Print and shaded views of the part. All mm, measured from the part's lowest x, y and z. A direction names the side the tool comes from. Coordinates: 2 decimals unless noted, no trailing zeros. Loops run counter-clockwise (first coordinate to the right, second up) from the corner with the lowest first, then second, coordinate; pieces in that order, holes last. Notation, with made-up numbers: M 17,65.5 L 23,65.5 A20 cw 23,98.5 Z; hole C 44,30.5 d6. An arc over 180 degrees is marked long. Answer as CSV lines item,"result". Start each with the question number.
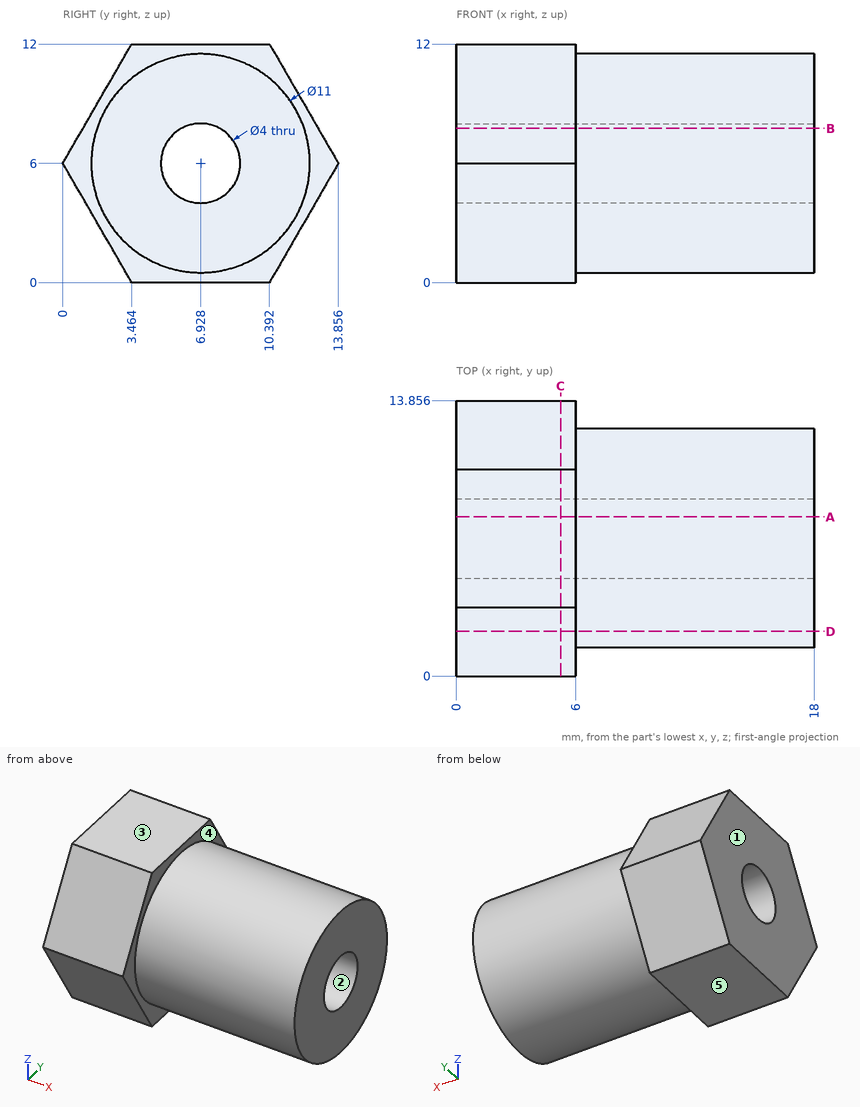
Q1. Two-plate mould, pull along Z, no slides. Class the marked faces 1, 2 and 3: +Z half, -Z half, draft (parallel to the pull), parting line (faces both ways), or undercut.
Q2. Wall check: L1, parallel to Y at x = 12.5, z = 6; L2, parallel to X at y = 12.75, z = 5.25; L3, parallel to Z at x = 10.5, y = 5.75 (1 decimal). Give the ranges that are in metal, low to high.
Q3. Flat gauge pins, fed straight in: P1, Ø3.5, axis at y = 6.93, z = 6, coming from the +X side; P2, Ø6, axis at x = 11.5, y = 11.5, coming from the -Z side; P3, Ø2, axis at x = 8, y = 7.5, coming from the -Z side. Where does each tip first touch, or does it go through?
Q4. Tool access for the marked faces 4 and 5: list every direction of +Z, -Z, +X, -X, +Y, -Y with a clear straight run to the whole face (end or side of a thin tool).
Q5. Slice it at C-C, the plane x = 5.25. Write the cut outline in (y, z).
Q6. Slice it at B-B, the plane z = 7.75. Write the cut outline in (x, y), and give its area (3 significant figures).
Q7. Slice it at D-D, the plane y = 2.25. Write the cut outline in (x, z).
Q8. Slice it at A-A, the plane y = 8. Write the cut outline in (x, z) (1 decimal), and give its area (3 significant figures).
Solved:
1,face 1,"draft"
1,face 2,"undercut"
1,face 3,"+Z half"
2,L1,"y = 1.43 to 4.93, 8.93 to 12.43"
2,L2,"x = 0 to 6"
2,L3,"z = 0.6 to 4.4, 7.6 to 11.4"
3,P1,"passes through"
3,P2,"stops at z = 0.73"
3,P3,"stops at z = 0.5"
4,face 4,"+X"
4,face 5,"-Z, +X, -X, +Y, -Y"
5,outline,"M 0,6 L 3.46,0 L 10.39,0 L 13.86,6 L 10.39,12 L 3.46,12 Z; hole C 6.93,6 d4"
6,outline,"M 0,1.01 L 6,1.01 L 6,1.71 L 18,1.71 L 18,5.96 L 0,5.96 Z; M 0,7.9 L 18,7.9 L 18,12.14 L 6,12.14 L 6,12.85 L 0,12.85 Z"
6,area,"161 mm2"
7,outline,"M 0,2.1 L 6,2.1 L 6,3.11 L 18,3.11 L 18,8.89 L 6,8.89 L 6,9.9 L 0,9.9 Z"
8,outline,"M 0,0 L 6,0 L 6,0.6 L 18,0.6 L 18,4.3 L 0,4.3 Z; M 0,7.7 L 18,7.7 L 18,11.4 L 6,11.4 L 6,12 L 0,12 Z"
8,area,"141 mm2"
